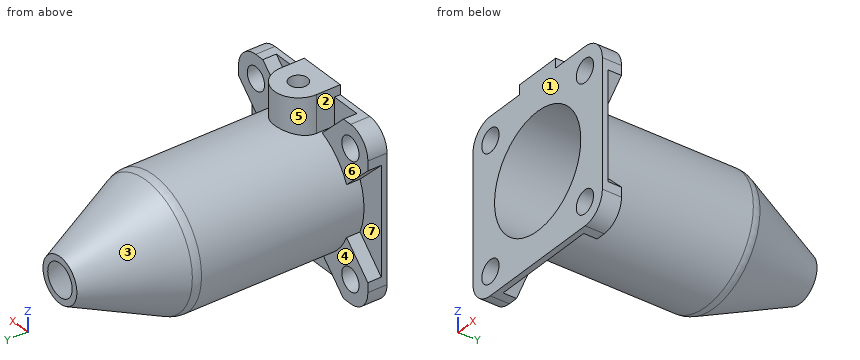
```python
from build123d import *

# Parameters (mm, degrees)
BOSS_EXTRUDE1_DEPTH = 3
SKETCH2_R           = 30
CUT_EXTRUDE1_DEPTH  = 3
BOSS_EXTRUDE2_DEPTH = 7
SKETCH5_R           = 6
CUT_EXTRUDE2_DEPTH  = 10
CIRPATTERN1_COUNT   = 4
BOSS_EXTRUDE3_START = -14.459044
BOSS_EXTRUDE3_DEPTH = 19.459044
SKETCH8_R           = 4.725
CUT_EXTRUDE3_DEPTH  = 18
FILLET1_R           = 10


with BuildPart() as part:
    # Sketch1 → Boss-Extrude1 (new body)
    with BuildSketch(Plane(origin=(0, 0, 0), x_dir=(1, 0, 0), z_dir=(0, 1, 0))):
        with BuildLine():
            Line((-33, -45), (33, -45))
            ThreePointArc((33, -45), (41.485281374, -41.485281374), (45, -33))
            Line((45, -33), (45, 33))
            ThreePointArc((45, 33), (41.485281374, 41.485281374), (33, 45))
            Line((33, 45), (-33, 45))
            ThreePointArc((-33, 45), (-41.485281374, 41.485281374), (-45, 33))
            Line((-45, 33), (-45, -33))
            ThreePointArc((-45, -33), (-41.485281374, -41.485281374), (-33, -45))
        make_face()
    extrude(amount=BOSS_EXTRUDE1_DEPTH)

    # Sketch2 → Cut-Extrude1 (cut)
    with BuildSketch(Plane(origin=(0, 3, 0), x_dir=(1, 0, 0), z_dir=(0, 1, 0))):
        with Locations(Location((0, 0, 0), (0, 0, 270))):
            Circle(SKETCH2_R)
    extrude(amount=-CUT_EXTRUDE1_DEPTH, mode=Mode.SUBTRACT)

    # Sketch3 → Revolve1 (revolve)
    with BuildSketch(Plane.XY, mode=Mode.PRIVATE) as revolve1_sk:
        Polygon((30, 3), (30, 89.354466715), (8.5, 137), (11.79129626, 137), (33, 90), (33, 3), align=None)
    revolve(revolve1_sk.sketch.rotate(Axis((0, -84.852813742, 0), (0, 1, 0)), 90), axis=Axis((0, -84.852813742, 0), (0, 1, 0)))

    # Sketch4 → Boss-Extrude2 (add)
    with BuildSketch(Plane(origin=(0, 3, 0), x_dir=(1, 0, 0), z_dir=(0, 1, 0))):
        with BuildLine():
            Line((-13.251783745, -30.222346494), (-28.029437252, -45))
            Line((-28.029437252, -45), (-33, -45))
            ThreePointArc((-33, -45), (-41.485281374, -41.485281374), (-45, -33))
            Line((-45, -33), (-45, -28.029437252))
            Line((-45, -28.029437252), (-30.222346494, -13.251783745))
            ThreePointArc((-30.222346494, -13.251783745), (-23.334523779, -23.334523779), (-13.251783745, -30.222346494))
        make_face()
    boss_extrude2 = extrude(amount=BOSS_EXTRUDE2_DEPTH)

    # Sketch5 → Cut-Extrude2 (cut)
    with BuildSketch(Plane(origin=(0, 10, 0), x_dir=(1, 0, 0), z_dir=(0, 1, 0))):
        with Locations(Location((-32.880465325, -32.880465325, 0), (0, 0, 270))):
            Circle(SKETCH5_R)
    cut_extrude2 = extrude(amount=-CUT_EXTRUDE2_DEPTH, mode=Mode.SUBTRACT)

    # CirPattern1: Boss-Extrude2, Cut-Extrude2 ×4 about axis
    cirpattern1_axis = Axis((0, 0, 0), (0, 1, 0))
    add([boss_extrude2.rotate(cirpattern1_axis, i * 360 / CIRPATTERN1_COUNT) for i in range(1, CIRPATTERN1_COUNT)])
    add([cut_extrude2.rotate(cirpattern1_axis, i * 360 / CIRPATTERN1_COUNT) for i in range(1, CIRPATTERN1_COUNT)], mode=Mode.SUBTRACT)

    # Sketch6 → Boss-Extrude3 (add)
    with BuildSketch(Plane.XY.offset(45).offset(BOSS_EXTRUDE3_START)):
        with BuildLine():
            Line((-12.5, 12.5), (-12.5, 0))
            Line((-12.5, 0), (12.5, 0))
            Line((12.5, 0), (12.5, 12.5))
            ThreePointArc((12.5, 12.5), (0, 25), (-12.5, 12.5))
        make_face()
    extrude(amount=BOSS_EXTRUDE3_DEPTH)

    # Sketch8 → Cut-Extrude3 (cut)
    with BuildSketch(Plane.XY.offset(50)):
        with Locations((0, 12.5)):
            Circle(SKETCH8_R)
    extrude(amount=-CUT_EXTRUDE3_DEPTH, mode=Mode.SUBTRACT)

    # Fillet1
    fillet1_edges = [part.edges().sort_by_distance(p)[0] for p in [
        (0, 90, 33),
    ]]
    fillet(fillet1_edges, radius=FILLET1_R)


solid = part.part
```
The listing builds one solid part. Answer for the finished solid, in the listing's coordinates (mm). Face numbers are marked on the shaded views. A direction names the side the tool comes from. Give positions to 0.01 mm unless a question says otherwise; leave off trailing zeros. Write each loop counter-clockwise with the first axis right and the second up, starting at its lowest first coordinate (ties: lowest second). Pieces come first, ordered by that corner, then holes. Notation, with made-up numbers: M 77,-34.75 L 103,-34.75 A22 cw 103,-16.75 Z; hole C 22,-13 d9. An arc over 180 degrees is marked long. Write each question's results on one line, items separated by ' | '.
Q1. Section B-B, the plane y = 28 is taken. Write down the section's boundary in (x, z).
Output values:
outline: C 0,0 d66; hole C 0,0 d60
Q2. Section A-A, the plane z = 36 is taken. Write down the section's boundary in (x, y) (3 decimals), then the cut area to 3 significant figures.
Output values:
outline: M -44.619,0 L -38.006,0 L -38.006,10 L -44.619,10 Z; M -27.755,0 L 27.755,0 L 27.755,10 L 19.029,10 L 19.029,3 L 12.5,3 L 12.5,12.5 A12.5 ccw -12.5,12.5 L -12.5,3 L -19.029,3 L -19.029,10 L -27.755,10 Z; M 38.006,0 L 44.619,0 L 44.619,10 L 38.006,10 Z; hole C 0,12.5 d9.45 | area: 834 mm2
Q3. Consider L1, parallel to Y at x = 32.5, z = -18; L2, parallel to Z at x = 6, y = 89.5; L3, parallel to X at y = 54, z = 0.5. Determine where each line is inside the solid, lowest interval first. Write a range as from..to.
Output values:
L1: 0..10 | L2: -32.31..-29.33, 29.33..32.31 | L3: -33..-30, 30..33
Q4. A tool of negligible diameter and unlimited length cuts with its end or side. For the marked faces 4, 5, 6 and 7, from which of +Z, -Z, +X, -X, +Y, -Y can it reach the whole face along a straight path? Write none if from no direction.
Output values:
face 4: -Z, -X, +Y | face 5: +Z, +Y | face 6: +Z, -X, +Y | face 7: -X, +Y
Q5. Flat-ended cylindrical pins translate along their axes: P1, Ø8, axis at x = -14, z = 4, coming from the -Y side; P2, Ø10, axis at x = -24.5, z = -5, coming from the +Y side; P3, Ø9.5, axis at x = 25, z = 24.5, coming from the +Y side; P4, Ø12.5, axis at x = 0, y = 12.5, coming from the +Z side. Find the tip coordinate at first contact, or state that the pin passes through.
Output values:
P1: y = 114.71 | P2: y = 118.8 | P3: y = 96.09 | P4: z = 50
Q6. For a pull along X with two mould halves and no side action, classify the marked faces 1, 2 and 3 as released by +X, released by -X, zero draft, split by the parting line, or undercut.
Output values:
face 1: zero draft | face 2: undercut | face 3: split by the parting line
Q7. Section C-C, the plane y = 94 is taken. Write down the section's boundary in (x, z) (3 decimals), then the cut area to 3 significant figures.
Output values:
outline: C 0,0 d62.39; hole C 0,0 d55.807 | area: 611 mm2
